Part model, mm, in its own coordinate system. A direction names the side the tool comes from. Coordinates: 2 decimals unless noted, no trailing zeros. Order: outer loops, then holes, each group sorted by start corner. A loop starts at its lowest first (then second) coordinate and runs counter-clockwise, first axis right, second up.
Autodesk Inventor part; units mm, degrees
ref_plane "Work Plane1" through (29, 0, 0) normal (0, -1, 0) x (1, 0, 0)
ref_plane "YZ Plane" through (0, 0, 0) normal (1, 0, 0) x (0, 1, 0)
ref_plane "XZ Plane" through (0, 0, 0) normal (0, 1, 0) x (-1, 0, 0)
sketch "Sketch1" plane through (0, 0, 0) normal (0, 0, 1) x (1, 0, 0)
  line L0 (-1.8333, 0) -> (25, 0)
  line L1 (25, 0) -> (25, 5)
  line L2 (25, 5) -> (4.5, 5)
  line L3 (4.5, 5) -> (3.5797, 5)
  line L4 (3.5797, 5) -> (0, 5)
  line L5 (0, 5) -> (0, 8)
  line L6 (0, 8) -> (-10, 8)
  line L7 (-10, 8) -> (-10, 4.6188)
  line L8 (-10, 4.6188) -> (-4.5, 4.6188)
  line L9 (-4.5, 4.6188) -> (-1.8333, 0)
  line L10 (-17, 0) -> (32, 0)
  line L11 (0, -1.6) -> (0, 9.6)
  line L12 (4.5, 5) -> (0, 5) construction
  dimension "d1" = 20.5
  dimension "d2" = 0.9203
  dimension "d3" = 10
  dimension "d4" = 5.5
  dimension "d5" = 60
  dimension "d6" = 10
  dimension "d7" = 10
  dimension "d8" = 9.2376
  dimension "d9" = 16
  dimension "d26" = 25
revolve "Body" add sketch "Sketch1" angle 360 about axis through (-1.8333, 0, 0) along (1, 0, 0)
sketch "Sketch2" plane through (-10, 0, 0) normal (-1, 0, 0) x (0, 0, 1)
  circle A0 centre (0, 0) radius 4.6188
  line L0 (0, -11.2) -> (0, 11.2)
  line L1 (-11.2, 0) -> (11.2, 0)
  line L2 (4.6188, 0) -> (2.3094, -4)
  line L3 (2.3094, -4) -> (-2.3094, -4)
  line L4 (-2.3094, -4) -> (-4.6188, 0)
  line L5 (-4.6188, 0) -> (-2.3094, 4)
  line L6 (-2.3094, 4) -> (2.3094, 4)
  line L7 (2.3094, 4) -> (4.6188, 0)
extrude "Slot" add sketch "Sketch2" against normal up to next contours L7 A0 | A0 L2 | L6 L0 A0 | A0 L0 L3 | L0 L6 A0 | A0 L3 L0 | L4 A0 | A0 L5
fillet "Fillet1" radius 1 1 edges at (-10, -8, 0)
thread "Thread"
chamfer "Chamfer1" distance 0.9202 distance2 0.9202 1 edges at (25, -5, 0) measured on face at (25, -0.8193, -0.3214)
ref_plane "Work Plane1" through (29, 0, 0) normal (0, -1, 0) x (1, 0, 0)
fillet "Fillet2" radius 0.1 1 edges at (0, -5, 0)
equation "\"d30\" = R"
equation "\"d17\" = RR"
equation "\"d13\" = GEL"
equation "\"d15\" = -0.5 * SPD + 0.5 * GD"
equation "\"d16\" = GUL"
equation "\"d1\" = GEL"
equation "\"d3\" = KOH"
equation "\"d4\" = INTI"
equation "\"d6\" = GD"
equation "\"d7\" = BDM"
equation "\"d8\" = 1.1547 * SW"
equation "\"d9\" = KOD"
equation "\"d26\" = NLG"
equation "\"GD\" = NND"
equation "\"NLG\" = 25"
equation "\"GEL\" = 20.5"
equation "\"KOD\" = 16"
equation "\"KOH\" = NND"
equation "\"INTI\" = 5.5"
equation "\"GAL\" = 0.61345 * PTC"
equation "\"GUL\" = 0.61345 * PTC"
equation "\"BDM\" = NND"
equation "\"SW\" = 8"
equation "\"RR\" = 1"
equation "\"SPD\" = NND - 1.2269 * PTC"
equation "\"R\" = 0.1"
equation "\"TOA\" = 30deg"
equation "\"GD1\" = THREADDIA - 1.2269 * PTC"
equation "\"FAWI\" = 45deg"
equation "\"PTC\" = 1.5"
equation "\"E0\" = 1.155 * SW"
equation "\"PHH\" = 0"
properties part number "CSN 02 1143 - M10 x 25" material "Steel, Mild"
Q1. Cut at A-A on x = 19. Write the cut outline in (y, z), and give its area (3 significant figures).
Results list:
outline: circle Ø10 at (0, 0)
area: 78.5 mm2
Q2. Pin check, flat tips, straight feed: pin 1 Ø2 at (y, z) = (-4, -4) entering from +X; pin 2 Ø8 at (x, y) = (-3, 5.5) entering from -Z; pin 3 Ø4 at (x, z) = (1.5, 2.5) entering from +Y. Stop position of each tip, or through.
Results list:
pin 1: stops at x = 24.42
pin 2: stops at z = -7.86
pin 3: stops at y = 7.91
Q3. Mould opens along Z. For faces 3 (the face through (11.92, -1.08, 4.88)), 4 (the face through (-7.11, 1.97, -3.48)), 5 (the face through (0, 5, -2)) say: pulls with the +Z half, pulls with the -Z half, needs draft (parallel to the pull), parting line crosses it, or undercut.
Results list:
face 3: parting line crosses it
face 4: undercut
face 5: needs draft
Q4. Wall check: line 1 along X through (y, z) = (5, 1.5); line 2 along Z through (x, y) = (-6, -0.25); line 3 along Z through (x, y) = (-4.5, 3.25). Give the ranges that are in metal, low to high.
Results list:
line 1: x = -10 to 0
line 2: z = -8 to -4.47, 4.47 to 8
line 3: z = -7.31 to -2.74, 2.74 to 7.31
Q5. Which spindle directions (+Z, -Z, +X, -X, +Y, -Y) get a long thin tool onto all of the face, cutting with end or side? Do faces 1 (the face through (-7, -4, 0)), 2 (the face through (-4.56, -1.73, 7.81)). Say none if no direction does.
Results list:
face 1: -X
face 2: +X, -X
